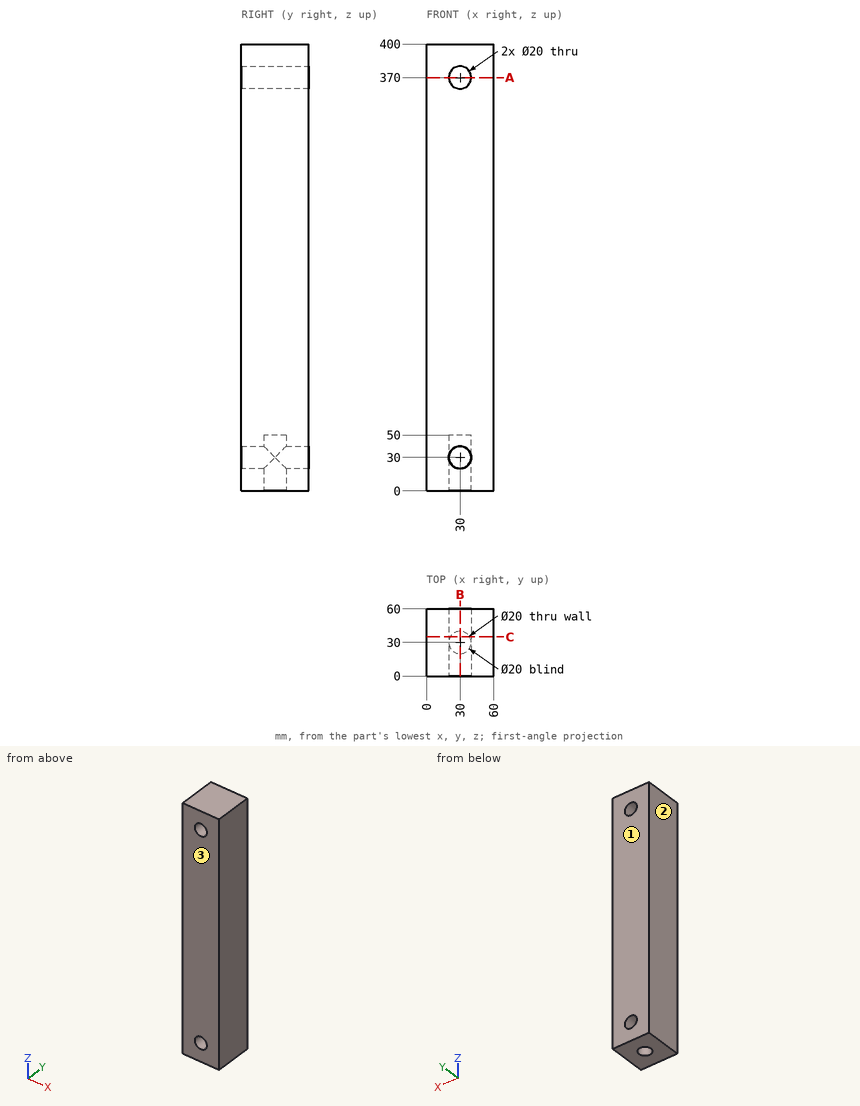
Could you check a few things on this drawing? It's one solid part, dimensions in mm from its lowest x, y, z. Coordinates: 2 decimals unless noted, no trailing zeros. Write each loop counter-clockwise with the first axis right and the second up, starting at its lowest first coordinate (ties: lowest second). Pieces come first, ordered by that corner, then holes. Notation, with made-up numbers: (3.25, -6.75) - (47.25, -6.75) arc R17 ccw to (47.25, 19.25) - close; hole circle Ø6 at (62.5, -30.75). An arc over 180 degrees is marked (long way). Use one line per item in the form item = value.
1) I'm going to push a flat-ended pin straight in: P1, Ø18, axis at x = 30, z = 30, coming from the +Y side. Where does the tip first touch, or does it pass through?
Solved:
P1 = through
2) I need wall thicknesses on line 1 (Z direction, x = 30, y = 42); line 2 (Y direction, x = 30, z = 40.5). Which ranges of each line are inside material? Lowest first, please.
Solved:
line_1 = 0 to 20, 40 to 360, 380 to 400
line_2 = 0 to 20, 40 to 60
3) Suppose I cut it at C-C, the plane y = 35. Write out the boundary of the cut face in (x, z), plus the area to 3 significant figures.
Solved:
outline = (0, 0) - (21.34, 0) - (21.34, 25) arc R10 cw to (21.34, 35) - (21.34, 50) - (38.66, 50) - (38.66, 35) arc R10 cw to (38.66, 25) - (38.66, 0) - (60, 0) - (60, 400) - (0, 400) - close; hole circle Ø20 at (30, 370)
area = 22,800 mm2
4) Suppose I cut it at B-B, the plane x = 30. Write out the boundary of the cut face in (y, z).
Solved:
outline = (0, 0) - (20, 0) - (20, 20) - (0, 20) - close; (0, 40) - (20, 40) - (20, 50) - (40, 50) - (40, 40) - (60, 40) - (60, 360) - (0, 360) - close; (0, 380) - (60, 380) - (60, 400) - (0, 400) - close; (40, 0) - (60, 0) - (60, 20) - (40, 20) - close
5) Suppose I cut it at A-A, the plane z = 370. Write out the boundary of the cut face in (x, y).
Solved:
outline = (0, 0) - (20, 0) - (20, 60) - (0, 60) - close; (40, 0) - (60, 0) - (60, 60) - (40, 60) - close
6) Thinking about a two-plate mould opening in Y: for the marked faces 1, 2 and 3, which applies, released by +Y, released by -Y, zero draft, split by the parting line, or undercut?
Solved:
face_1 = released by +Y
face_2 = zero draft
face_3 = released by -Y
